Part model, mm, in its own coordinate system. Face numbers are marked on the shaded views. A direction names the side the tool comes from. Round coordinates to 2 decimals unless told otherwise and drop trailing zeros. Order: outer loops, then holes, each group sorted by start corner. A loop starts at its lowest first (then second) coordinate and runs counter-clockwise, first axis right, second up. Notation, with made-up numbers: (-22, 18) - (-1, 18) arc R10 ccw to (-1, 27) - close; hole circle Ø8 at (37, 40). An arc over 180 degrees is marked (long way). Answer as a JSON object with one key per item and string values.
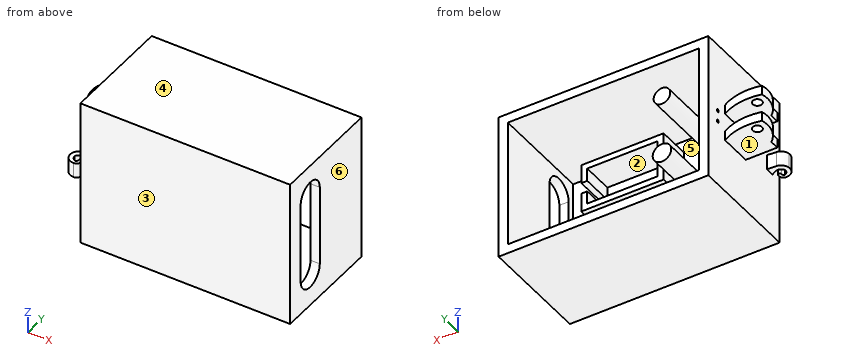
```python
from build123d import *

# Parameters (mm, degrees)
BOSS_EXTRUDE1_DEPTH     = 38.1
CUT_EXTRUDE1_DEPTH      = 34.925
SERVO_BOX_1_DEPTH       = 13.97
SERVO_BOX_2_DEPTH       = 13.97
SKETCH36_R              = 1.5875
RING_ATTACHMENT_DEPTH   = 19.05
ATTACHMENT_TRIM_DEPTH   = 25.4
SKETCH33_R              = 0.508
RING_FINGER_HOLES_DEPTH = 31.75
CORD_HOLE_DEPTH         = 44.45
RING_HOOK_DEPTH         = 19.05
MIDDLE_HOOK_DEPTH       = 19.05
MIDDLE_HOOK_2_DEPTH     = 19.05
SKETCH57_W              = 6.44385504
SKETCH57_H              = 7.30367128
MIDDLE_HOOK_CUT_1_DEPTH = 19.05
SKETCH65_W              = 5.804806401
SKETCH65_H              = 9.582838289
SKETCH65_H_2            = 6.985
SKETCH65_W_2            = 10.36865681
SKETCH65_H_3            = 26.914043033
CUT_EXTRUDE9_DEPTH      = 15.24
CUT_EXTRUDE10_DEPTH     = 50.8
SKETCH67_R              = 2.848989685
SKETCH67_R_2            = 3.175
BOSS_EXTRUDE2_DEPTH     = 38.1


with BuildPart() as part:
    # Sketch2 → Boss-Extrude1 (new body)
    with BuildSketch(Plane(origin=(0, 0, 0), x_dir=(1, 0, 0), z_dir=(0, 1, 0))):
        with BuildLine():
            Line((-20.778406205, 52.758673202), (-36.188953289, 52.758673202))
            Line((-36.188953289, 52.758673202), (-36.188953289, 33.708673202))
            Line((-36.188953289, 33.708673202), (-38.864171838, 27.358673202))
            Line((-38.864171838, 27.358673202), (-48.947687906, 27.358673202))
            Line((-48.947687906, 27.358673202), (-48.947687906, 8.308673202))
            Line((-48.947687906, 8.308673202), (-48.947687906, -42.491326798))
            Line((-48.947687906, -42.491326798), (-42.959403849, -42.491326798))
            ThreePointArc((-42.959403849, -42.491326798), (-29.448791922, -45.239401215), (-16.422067996, -49.755263412))
            ThreePointArc((-16.422067996, -49.755263412), (-10.441569813, -54.6928899), (-3.738179712, -58.593027718))
            Line((-3.738179712, -58.593027718), (-3.738179712, -63.210333869))
            Line((-3.738179712, -63.210333869), (15.311820288, -63.210333869))
            ThreePointArc((15.311820288, -63.210333869), (19.123708761, -63.010602415), (22.909801598, -62.524919994))
            Line((22.909801598, -62.524919994), (22.909801598, 48.896004027))
            ThreePointArc((22.909801598, 48.896004027), (1.17082788, 52.016399628), (-20.778406205, 52.758673202))
        make_face()
    extrude(amount=BOSS_EXTRUDE1_DEPTH)

    # Sketch3 → Cut-Extrude1 (cut)
    with BuildSketch(Plane(origin=(0, 38.1, 0), x_dir=(1, 0, 0), z_dir=(0, 1, 0))):
        Polygon((-45.772687906, 24.183673202), (19.734801598, 24.183673202), (19.734801598, -19.921590233), (-45.772687906, -19.921590233), (-45.772687906, 7.713042295), align=None)
        with BuildLine():
            Line((-38.864171838, 27.358673202), (22.909801598, 27.358673202))
            ThreePointArc((22.909801598, 27.358673202), (-7.97718512, 133.680362497), (-38.864171838, 27.358673202))
        make_face()
        with BuildLine():
            Line((-48.947687906, -23.096590233), (22.909801598, -23.096590233))
            ThreePointArc((22.909801598, -23.096590233), (35.616611998, -147.942668358), (-48.947687906, -55.22327753))
            Line((-48.947687906, -55.22327753), (-48.947687906, -23.096590233))
        make_face()
    extrude(amount=-CUT_EXTRUDE1_DEPTH, mode=Mode.SUBTRACT)

    # Sketch6 → Servo Box 1 (add)
    with BuildSketch(Plane(origin=(0, 0, 0), x_dir=(1, 0, 0), z_dir=(0, 1, 0))):
        Polygon((-18.154039747, -9.466732857), (-16.122039747, -9.466732857), (-16.122039747, -13.911732857), (8.007960253, -13.911732857), (8.007960253, -9.466732857), (10.039960253, -9.466732857), (10.039960253, -15.943732857), (-18.154039747, -15.943732857), align=None)
        Polygon((8.007960253, -1.211732857), (-16.122039747, -1.211732857), (-16.122039747, -5.656732857), (-18.154039747, -5.656732857), (-18.154039747, 0.820267143), (10.039960253, 0.820267143), (10.039960253, -5.656732857), (8.007960253, -5.656732857), align=None)
    extrude(amount=SERVO_BOX_1_DEPTH)

    # Sketch7 → Servo Box 2 (add)
    with BuildSketch(Plane(origin=(0, 0, 0), x_dir=(1, 0, 0), z_dir=(0, 1, 0))):
        Polygon((-18.154039747, 10.472267143), (-16.122039747, 10.472267143), (-16.122039747, 6.027267143), (8.007960253, 6.027267143), (8.007960253, 10.472267143), (10.039960253, 10.472267143), (10.039960253, 3.995267143), (-18.154039747, 3.995267143), align=None)
        Polygon((8.007960253, 18.727267143), (-16.122039747, 18.727267143), (-16.122039747, 14.282267143), (-18.154039747, 14.282267143), (-18.154039747, 20.759267143), (10.039960253, 20.759267143), (10.039960253, 14.282267143), (8.007960253, 14.282267143), align=None)
    extrude(amount=SERVO_BOX_2_DEPTH)

    # Sketch36 → Ring Attachment (add)
    with BuildSketch(Plane(origin=(0, 0, -12.118673202), x_dir=(-1, 0, 0), z_dir=(0, 0, -1))):
        with BuildLine():
            Line((48.947687906, 29.21), (48.947687906, 18.074207691))
            Line((48.947687906, 18.074207691), (53.392687906, 18.074207691))
            Line((53.392687906, 18.074207691), (59.742687906, 18.074207691))
            Line((59.742687906, 18.074207691), (59.742687906, 21.249207691))
            ThreePointArc((59.742687906, 21.249207691), (62.80538306, 25.776891551), (62.917687906, 31.242))
            ThreePointArc((62.917687906, 31.242), (55.737515168, 31.567812574), (48.947687906, 29.21))
        make_face()
        with Locations((59.742687906, 28.707395517)):
            Circle(SKETCH36_R, mode=Mode.SUBTRACT)
    extrude(amount=-RING_ATTACHMENT_DEPTH)

    # Sketch40 → Attachment Trim (cut)
    with BuildSketch(Plane(origin=(0, 38.1, 0), x_dir=(1, 0, 0), z_dir=(0, 1, 0))):
        with BuildLine():
            Line((-48.947687906, -6.931326798), (-48.947687906, -3.756326798))
            Line((-48.947687906, -3.756326798), (-65.361733155, -3.756326798))
            Line((-65.361733155, -3.756326798), (-65.361733155, -0.581326798))
            Line((-65.361733155, -0.581326798), (-48.947687906, -0.581326798))
            Line((-48.947687906, -0.581326798), (-48.947687906, 5.768673202))
            Line((-48.947687906, 5.768673202), (-65.776264763, 5.768673202))
            Line((-65.776264763, 5.768673202), (-65.776264763, 8.943673202))
            Line((-65.776264763, 8.943673202), (-48.947687906, 8.943673202))
            Line((-48.947687906, 8.943673202), (-48.947687906, 12.118673202))
            ThreePointArc((-48.947687906, 12.118673202), (-80.34840255, 2.593673202), (-48.947687906, -6.931326798))
        make_face()
    extrude(amount=-ATTACHMENT_TRIM_DEPTH, mode=Mode.SUBTRACT)

    # Sketch33 → Ring Finger Holes (cut)
    with BuildSketch(Plane(origin=(-69.85, 0, 0), x_dir=(0, 0, -1), z_dir=(1, 0, 0))):
        with Locations((0.688673202, 33.02)):
            Circle(SKETCH33_R)
        with Locations((4.498673202, 33.02)):
            Circle(SKETCH33_R)
    extrude(amount=RING_FINGER_HOLES_DEPTH, mode=Mode.SUBTRACT)

    # Sketch41 → Cord Hole (cut)
    with BuildSketch(Plane(origin=(62.913848002, 0, 0), x_dir=(0, 0, -1), z_dir=(1, 0, 0))):
        with BuildLine():
            Line((-12.016652412, 15.851932983), (15.710210154, 15.851932983))
            ThreePointArc((15.710210154, 15.851932983), (20.818250673, 10.743892464), (15.710210154, 5.635851946))
            Line((15.710210154, 5.635851946), (-12.016652412, 5.635851946))
            ThreePointArc((-12.016652412, 5.635851946), (-17.12469293, 10.743892464), (-12.016652412, 15.851932983))
        make_face()
    extrude(amount=-CORD_HOLE_DEPTH, mode=Mode.SUBTRACT)

    # Sketch52 → Ring Hook (add)
    with BuildSketch(Plane(origin=(0, 0, -12.118673202), x_dir=(-1, 0, 0), z_dir=(0, 0, -1))):
        with BuildLine():
            Line((52.079417812, 6.575838366), (48.947687906, 6.798773562))
            Line((48.947687906, 6.798773562), (48.947687906, 3.681759929))
            ThreePointArc((48.947687906, 3.681759929), (50.154592803, 4.494095024), (51.56202319, 4.862398487))
            ThreePointArc((51.56202319, 4.862398487), (52.595162873, 4.406515303), (53.259394348, 3.493277311))
            ThreePointArc((53.259394348, 3.493277311), (52.80871858, 2.435311228), (51.875495098, 1.763377592))
            ThreePointArc((51.875495098, 1.763377592), (51.337693114, 2.052625855), (51.280629769, 2.660605548))
            ThreePointArc((51.280629769, 2.660605548), (50.525041175, 3.111212192), (50.07443453, 2.355623598))
            ThreePointArc((50.07443453, 2.355623598), (50.521061084, 1.129253272), (51.719490009, 0.612312688))
            ThreePointArc((51.719490009, 0.612312688), (54.01907529, 1.640613281), (54.717115143, 4.060992371))
            ThreePointArc((54.717115143, 4.060992371), (53.825637568, 5.766663725), (52.079417812, 6.575838366))
        make_face()
    extrude(amount=-RING_HOOK_DEPTH)


with BuildPart() as body_2:
    # Sketch56 → Middle Hook (new body)
    with BuildSketch(Plane(origin=(0, 0, 13.281326798), x_dir=(-1, 0, 0), z_dir=(0, 0, -1))):
        with BuildLine():
            Line((59.307557511, 8.89), (56.767557511, 8.89))
            Line((56.767557511, 8.89), (56.767557511, 12.007013633))
            ThreePointArc((56.767557511, 12.007013633), (57.832492224, 10.713868099), (59.307557511, 9.919831756))
            ThreePointArc((59.307557511, 9.919831756), (60.589681431, 10.520271405), (61.228710278, 11.783604952))
            ThreePointArc((61.228710278, 11.783604952), (60.623886944, 13.07409489), (59.342790307, 13.69856823))
            ThreePointArc((59.342790307, 13.69856823), (58.957508965, 13.481176717), (58.80220943, 13.066951131))
            ThreePointArc((58.80220943, 13.066951131), (58.461789356, 12.706641867), (58.101480093, 13.047061941))
            ThreePointArc((58.101480093, 13.047061941), (58.440138088, 13.935120258), (59.307557511, 14.323604952))
            ThreePointArc((59.307557511, 14.323604952), (61.228626965, 13.52787193), (62.024359987, 11.606802476))
            ThreePointArc((62.024359987, 11.606802476), (61.228626965, 9.685733022), (59.307557511, 8.89))
        make_face()
    extrude(amount=-MIDDLE_HOOK_DEPTH)

    # Sketch57 → Middle Hook Cut 1 (cut)
    with BuildSketch(Plane(origin=(0, 0, 13.281326798), x_dir=(-1, 0, 0), z_dir=(0, 0, -1))):
        with Locations((59.989485031, 11.404925675)):
            Rectangle(SKETCH57_W, SKETCH57_H)
    extrude(amount=-MIDDLE_HOOK_CUT_1_DEPTH, mode=Mode.SUBTRACT)


with BuildPart() as body_3:
    # Sketch56 → Middle Hook 2 (new body)
    with BuildSketch(Plane(origin=(0, 0, 13.281326798), x_dir=(-1, 0, 0), z_dir=(0, 0, -1))):
        with BuildLine():
            Line((59.307557511, 6.798773562), (56.767557511, 6.798773562))
            Line((56.767557511, 6.798773562), (56.767557511, 3.681759929))
            ThreePointArc((56.767557511, 3.681759929), (57.832492224, 4.974905464), (59.307557511, 5.768941806))
            ThreePointArc((59.307557511, 5.768941806), (60.589681431, 5.168502157), (61.228710278, 3.905168611))
            ThreePointArc((61.228710278, 3.905168611), (60.623886944, 2.614678673), (59.342790307, 1.990205333))
            ThreePointArc((59.342790307, 1.990205333), (58.957508965, 2.207596845), (58.80220943, 2.621822432))
            ThreePointArc((58.80220943, 2.621822432), (58.461789356, 2.982131695), (58.101480093, 2.641711621))
            ThreePointArc((58.101480093, 2.641711621), (58.440138088, 1.753653304), (59.307557511, 1.365168611))
            ThreePointArc((59.307557511, 1.365168611), (61.228626965, 2.160901633), (62.024359987, 4.081971086))
            ThreePointArc((62.024359987, 4.081971086), (61.228626965, 6.00304054), (59.307557511, 6.798773562))
        make_face()
    extrude(amount=-MIDDLE_HOOK_2_DEPTH)


with BuildPart() as cut_extrude9_tool:
    # Sketch65 → Cut-Extrude9 (new body)
    with BuildSketch(Plane(origin=(0, 0, 0), x_dir=(1, 0, 0), z_dir=(0, 1, 0))):
        with Locations((-51.850091107, 9.925092347)):
            Rectangle(SKETCH65_W, SKETCH65_H)
        with Locations((-51.850091107, -3.438826798)):
            Rectangle(SKETCH65_W, SKETCH65_H_2)
        with Locations((-59.388818787, -23.035181565)):
            Rectangle(SKETCH65_W_2, SKETCH65_H_3)
    extrude(amount=CUT_EXTRUDE9_DEPTH)


with BuildPart() as part_1:
    add(part.part)

    # Cut-Extrude9: cut by cut_extrude9_tool
    add(cut_extrude9_tool.part, mode=Mode.SUBTRACT)

    # Sketch66 → Cut-Extrude10 (cut)
    with BuildSketch(Plane(origin=(0, 38.1, 0), x_dir=(1, 0, 0), z_dir=(0, 1, 0))):
        with BuildLine():
            Line((-48.947687906, -23.096590233), (22.909801598, -23.096590233))
            ThreePointArc((22.909801598, -23.096590233), (-13.018943154, -212.453183119), (-48.947687906, -23.096590233))
        make_face()
        with BuildLine():
            Line((22.909801598, 27.358673202), (-48.947687906, 27.358673202))
            ThreePointArc((-48.947687906, 27.358673202), (-13.018943154, 126.14838829), (22.909801598, 27.358673202))
        make_face()
    extrude(amount=-CUT_EXTRUDE10_DEPTH, mode=Mode.SUBTRACT)

    # Sketch67 → Boss-Extrude2 (add)
    with BuildSketch(Plane(origin=(0, 38.1, 0), x_dir=(1, 0, 0), z_dir=(0, 1, 0))):
        with Locations((-33.072687906, -7.879232857)):
            Circle(SKETCH67_R)
        with Locations((-33.072687906, 12.694767143)):
            Circle(SKETCH67_R_2)
    extrude(amount=-BOSS_EXTRUDE2_DEPTH)


with BuildPart() as body_3_1:
    add(body_3.part)

    # Cut-Extrude9: cut by cut_extrude9_tool
    add(cut_extrude9_tool.part, mode=Mode.SUBTRACT)


solid = part_1.part
```
Item 1: Tool access for the marked faces 1, 2 and 3: list every direction of +Z, -Z, +X, -X, +Y, -Y with a clear straight run to the whole face (end or side of a thin tool).
Taken from the geometry:
{"face 1": "-Z, -X, +Y, -Y", "face 2": "+Y", "face 3": "+Z, -Z, +X, -X, -Y"}
Item 2: Two-plate mould, pull along X, no slides. Class the marked faces 4, 5 and 6: pulls with the +X half, pulls with the -X half, needs draft (parallel to the pull), parting line crosses it, or undercut.
Taken from the geometry:
{"face 4": "needs draft", "face 5": "undercut", "face 6": "pulls with the +X half"}
Item 3: Probe L1, parallel to Z at x = -47.5, y = 33.02; L2, parallel to Z at x = -15.5, y = 5; L3, parallel to X at y = 12.5, z = -7. List the from-to ranges inside material, lowest first. Write a range as from..to.
Taken from the geometry:
{"L1": "-27.36..-5.01, -3.99..-1.2, -0.18..23.1", "L2": "-27.36..-24.18, -20.76..-18.73, -6.03..-4, -0.82..1.21, 13.91..15.94, 19.92..23.1", "L3": "-48.95..-45.77, -18.15..-16.12, 8.01..10.04"}
Item 4: Cut at C-C (x = -2.5). Write the cut outline in (y, z) (3 decimals).
Taken from the geometry:
{"outline": "(0, -27.359) - (38.1, -27.359) - (38.1, -24.184) - (3.175, -24.184) - (3.175, -20.759) - (13.97, -20.759) - (13.97, -18.727) - (3.175, -18.727) - (3.175, -6.027) - (13.97, -6.027) - (13.97, -3.995) - (3.175, -3.995) - (3.175, -0.82) - (13.97, -0.82) - (13.97, 1.212) - (3.175, 1.212) - (3.175, 13.912) - (13.97, 13.912) - (13.97, 15.944) - (3.175, 15.944) - (3.175, 19.922) - (38.1, 19.922) - (38.1, 23.097) - (0, 23.097) - close"}
Item 5: Drop flat-ended pins along their axis: P1, Ø10, axis at y = 14, z = 8.5, coming from the +X side; P2, Ø7, axis at x = 0, z = 2.5, coming from the +Y side; P3, Ø6, axis at y = 5, z = 14, coming from the -X side; P4, Ø3, axis at x = -8, z = 12, coming from the +Y side (3 decimals). Give the stop position or say it passes through.
Taken from the geometry:
{"P1": "x = 22.91", "P2": "y = 13.97", "P3": "x = -48.95", "P4": "y = 3.175"}
Item 6: Cut at D-D (y = 23.5). Write the cut outline in (x, z) (3 decimals).
Taken from the geometry:
{"outline": "(-61.738, -8.944) - (-48.948, -8.944) - (-48.948, -27.359) - (22.91, -27.359) - (22.91, 23.097) - (-48.948, 23.097) - (-48.948, 3.756) - (-61.738, 3.756) - (-61.738, 0.581) - (-48.948, 0.581) - (-48.948, -5.769) - (-61.738, -5.769) - close; circle Ø6.35 at (-33.073, -12.695); circle Ø5.698 at (-33.073, 7.879); hole (-45.773, -24.184) - (19.735, -24.184) - (19.735, 19.922) - (-45.773, 19.922) - close"}
Item 7: Cut at A-A (y = 19). Write the cut outline in (x, z) (3 decimals).
Taken from the geometry:
{"outline": "(-59.743, -8.944) - (-48.948, -8.944) - (-48.948, -27.359) - (22.91, -27.359) - (22.91, 23.097) - (-48.948, 23.097) - (-48.948, 3.756) - (-59.743, 3.756) - (-59.743, 0.581) - (-48.948, 0.581) - (-48.948, -5.769) - (-59.743, -5.769) - close; circle Ø6.35 at (-33.073, -12.695); circle Ø5.698 at (-33.073, 7.879); hole (-45.773, -24.184) - (19.735, -24.184) - (19.735, 19.922) - (-45.773, 19.922) - close"}
Item 8: Cut at B-B (z = -7). State how many separate pieces and enclosed holes the cut face has, plus the area to 3 significant figures.
Taken from the geometry:
{"separate pieces": "2", "enclosed holes": "1", "area": "621 mm2"}
